Autodesk Inventor part; units mm, degrees
ref_plane "YZ Plane" through (0, 0, 0) normal (1, 0, 0) x (0, 1, 0)
ref_plane "XZ Plane" through (0, 0, 0) normal (0, 1, 0) x (-1, 0, 0)
ref_plane "XY Plane" through (0, 0, 0) normal (0, 0, 1) x (1, 0, 0)
sketch "Sketch1" plane through (0, 0, 0) normal (0, 0, 1) x (1, 0, 0)
  circle A0 centre (0, 0) radius 8.15
  dimension "d0" = 16.3
extrude "Extrusion1" add sketch "Sketch1" along normal blind 12
sketch "Sketch2" plane through (0, 0, 12) normal (0, 0, 1) x (1, 0, 0)
  circle A0 centre (0, 0) radius 8.15
hole "Hole1" at (0, 0, 12) direction (0, 0, -1) diameter 13 depth 0.5
fillet "Fillet1" radius 0.5 2 edges at (-8.15, 0, 12) (0, 6.5, 12)
properties part number "Parallax_Ping_Transducer" material "ABS Plastic"
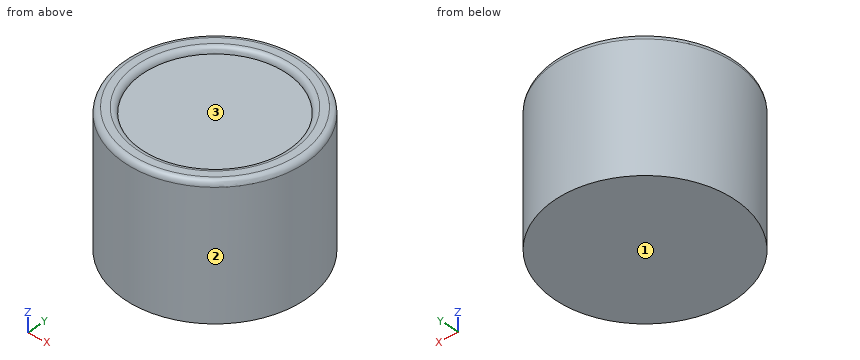
Source: CAD feature listing. Evaluate the final solid. Frame: model axes, mm. Face numbers are marked on the shaded views. Round coordinates to 2 decimals unless told otherwise and drop trailing zeros. Loops run counter-clockwise (first coordinate to the right, second up) from the corner with the lowest first, then second, coordinate; pieces in that order, holes last. Notation, with made-up numbers: (76.25, 73) - (90.25, 73) arc R18 cw to (90.25, 90) - close; hole circle Ø2 at (-12, -31.5). An arc over 180 degrees is marked (long way). Write item = value, one per line. Start each with the question number.
Item 1: First-contact query: pin 1 Ø5 at (y, z) = (5, 4) entering from -X; pin 2 Ø1.5 at (x, y) = (-1, 3.5) entering from +Z; pin 3 Ø6 at (x, z) = (5, 4.5) entering from -Y. Flat tips, straight axial feed; report the tip coordinate or a pass-through.
Item 2: Material intervals for line 1 (Z direction, x = 2.75, y = 4.25); line 2 (Y direction, x = 0, z = 11.55); line 3 (X direction, y = -0.25, z = 2.5), sorted ascending.
Item 3: Mould query, pull axis X, two halves, no side actions, for the marked faces 1, 2 and 3. Classes: released by +X, released by -X, zero draft, split by the parting line, or undercut.
Item 4: Section query C-C on z = 7.25. Output: boundary loops of the cut face in (x, y), plus the area to 3 significant figures.
Results list:
q1.pin_1 = -7.76
q1.pin_2 = 11.5
q1.pin_3 = -7.9
q2.line_1 = 0 to 11.5
q2.line_2 = -8.15 to -6.5, 6.5 to 8.15
q2.line_3 = -8.15 to 8.15
q3.face_1 = zero draft
q3.face_2 = split by the parting line
q3.face_3 = undercut
q4.outline = circle Ø16.3 at (0, 0)
q4.area = 209 mm²
